Work out the finished part from the listing and answer in its coordinate system (mm). A direction names the side the tool comes from. Give positions to 0.01 mm unless a question says otherwise; leave off trailing zeros. Order: outer loops, then holes, each group sorted by start corner. A loop starts at its lowest first (then second) coordinate and runs counter-clockwise, first axis right, second up. Notation, with made-up numbers: (1, 0) - (6, 0) arc R12 ccw to (6, 16) - close; hole circle Ø1 at (-2, -1). An arc over 180 degrees is marked (long way). Write each question's results on one line, items separated by ' | '.
from build123d import *

# Parameters (mm, degrees)
SKETCH1_W                                       = 55
SKETCH1_H                                       = 55
BOSS_EXTRUDE1_DEPTH                             = 5
SKETCH2_W                                       = 5
SKETCH2_H                                       = 55
BOSS_EXTRUDE2_DEPTH                             = 47.3
CUT_EXTRUDE1_REACH                              = 54.3
SKETCH3_R                                       = 16.5
SKETCH4_W                                       = 5
SKETCH4_H                                       = 55
BOSS_EXTRUDE3_DEPTH                             = 20
SKETCH5_W                                       = 5
SKETCH5_H                                       = 55
BOSS_EXTRUDE4_DEPTH                             = 20
CSK_FOR_M2_FLAT_HEAD_MACHINE_SCREW1_D           = 2.4
CSK_FOR_M2_FLAT_HEAD_MACHINE_SCREW1_CSINK_D     = 4.4
CSK_FOR_M2_FLAT_HEAD_MACHINE_SCREW1_CSINK_ANGLE = 90


with BuildPart() as part:
    # Sketch1 → Boss-Extrude1 (new body)
    with BuildSketch(Plane.XY):
        Rectangle(SKETCH1_W, SKETCH1_H)
    extrude(amount=BOSS_EXTRUDE1_DEPTH)

    # Sketch2 → Boss-Extrude2 (add)
    with BuildSketch(Plane(origin=(0, 0, 0), x_dir=(-1, 0, 0), z_dir=(0, 0, -1))):
        with Locations((-25, 0)):
            Rectangle(SKETCH2_W, SKETCH2_H)
        with Locations((25, 0)):
            Rectangle(SKETCH2_W, SKETCH2_H)
    extrude(amount=BOSS_EXTRUDE2_DEPTH)

    # Sketch3 → Cut-Extrude1 (cut, up to next)
    with BuildSketch(Plane.XY.offset(5), mode=Mode.PRIVATE) as cut_extrude1_sk1:
        Circle(SKETCH3_R)
    cut_extrude1_tool1 = extrude(cut_extrude1_sk1.sketch, amount=-CUT_EXTRUDE1_REACH, mode=Mode.PRIVATE) & part.part
    add(cut_extrude1_tool1.solids().sort_by_distance((0, 0, 5))[0], mode=Mode.SUBTRACT)

    # Sketch4 → Boss-Extrude3 (add)
    with BuildSketch(Plane(origin=(27.5, 0, 0), x_dir=(0, 0, -1), z_dir=(1, 0, 0))):
        with Locations((44.8, 0)):
            Rectangle(SKETCH4_W, SKETCH4_H)
    extrude(amount=BOSS_EXTRUDE3_DEPTH)

    # Sketch5 → Boss-Extrude4 (add)
    with BuildSketch(Plane.ZY.offset(27.5)):
        with Locations((-44.8, 0)):
            Rectangle(SKETCH5_W, SKETCH5_H)
    extrude(amount=BOSS_EXTRUDE4_DEPTH)

    # CSK for M2 Flat Head Machine Screw1 (through all)
    with Locations(Plane.XY.offset(-42.3)):
        with Locations((-37.5, 15.5), (-37.5, -15.5), (37.5, 15.5), (37.5, -15.5)):
            CounterSinkHole(CSK_FOR_M2_FLAT_HEAD_MACHINE_SCREW1_D / 2, CSK_FOR_M2_FLAT_HEAD_MACHINE_SCREW1_CSINK_D / 2, counter_sink_angle=CSK_FOR_M2_FLAT_HEAD_MACHINE_SCREW1_CSINK_ANGLE)


solid = part.part
1. Given P1, Ø1, axis at y = -8, z = -19, coming from the +X side; P2, Ø1.4, axis at x = 37.5, y = 15.5, coming from the +Z side; P3, Ø3, axis at x = -31, y = -8, coming from the +Z side; P4, Ø10, axis at y = -16.5, z = -7, coming from the -X side, each flat-ended and moving along its own axis, determine where each tip first touches the part or whether it passes through.
Answer list:
P1: x = 27.5 | P2: through | P3: z = -42.3 | P4: x = -27.5
2. A cutting plane is placed at B-B, the plane x = 0. Write down the section's boundary in (y, z), then the cut area to 3 significant figures.
Answer list:
outline: (-27.5, 0) - (-16.5, 0) - (-16.5, 5) - (-27.5, 5) - close; (16.5, 0) - (27.5, 0) - (27.5, 5) - (16.5, 5) - close | area: 110 mm^2
3. A cutting plane is placed at D-D, the plane y = -23. Write down the section's boundary in (x, z).
Answer list:
outline: (-47.5, -47.3) - (-22.5, -47.3) - (-22.5, 0) - (22.5, 0) - (22.5, -47.3) - (47.5, -47.3) - (47.5, -42.3) - (27.5, -42.3) - (27.5, 5) - (-27.5, 5) - (-27.5, -42.3) - (-47.5, -42.3) - close
4. A cutting plane is placed at A-A, the plane x = 37.5. Write down the section's boundary in (y, z).
Answer list:
outline: (-27.5, -47.3) - (-16.7, -47.3) - (-16.7, -43.3) - (-17.7, -42.3) - (-27.5, -42.3) - close; (-14.3, -47.3) - (14.3, -47.3) - (14.3, -43.3) - (13.3, -42.3) - (-13.3, -42.3) - (-14.3, -43.3) - close; (16.7, -47.3) - (27.5, -47.3) - (27.5, -42.3) - (17.7, -42.3) - (16.7, -43.3) - close
5. Straight lines are drawn through the part: line 1 (Y direction, x = 37.5, z = -44.3); line 2 (X direction, y = -23, z = -33); line 3 (X direction, y = 15.5, z = -46). For each, find the intervals that lie inside material, in ascending order. Write a range as [from, to].
Answer list:
line 1: [-27.5, -16.7], [-14.3, 14.3], [16.7, 27.5] | line 2: [-27.5, -22.5], [22.5, 27.5] | line 3: [-47.5, -38.7], [-36.3, -22.5], [22.5, 36.3], [38.7, 47.5]
6. Determine the mould class of faces 4 (the face through (36.39, -15.96, -45.33)), 5 (the face through (-27.5, 0, -19)), 6 (the face through (0, -27.5, 2)) for opening direction Y: +Y half, -Y half, draft (parallel to the pull), parting line (faces both ways), or undercut.
Answer list:
face 4: undercut | face 5: draft | face 6: -Y half
7. A cutting plane is placed at C-C, the plane z = -31. Write down the section's boundary in (x, y), then the cut area to 3 significant figures.
Answer list:
outline: (-27.5, -27.5) - (-22.5, -27.5) - (-22.5, 27.5) - (-27.5, 27.5) - close; (22.5, -27.5) - (27.5, -27.5) - (27.5, 27.5) - (22.5, 27.5) - close | area: 550 mm^2
8. A tool of negligible diameter and unlimited length cuts with its end or side. For faces 1 (the face through (22.5, 0, -23)), 2 (the face through (-37, 0, -42.3)), 3 (the face through (27.5, 0, -18)), from which of +Z, -Z, +X, -X, +Y, -Y can it reach the whole face along a straight path? Write none if from no direction.
Answer list:
face 1: -Z, +Y, -Y | face 2: +Z, -X, +Y, -Y | face 3: +Z, +X, +Y, -Y
